from build123d import *

# Parameters (mm, degrees)
EXTRUDE_1_DEPTH              = 4
HOLE_WIZARD_M5_1_D           = 8
HOLE_WIZARD_M5_1_DEPTH       = 12.4
HOLE_WIZARD_M5_1_CBORE_D     = 9.5
HOLE_WIZARD_M5_1_CBORE_DEPTH = 0.9
HOLE_WIZARD_M5_1_TIP         = 2.403442476
SKETCH_4_R                   = 1.5
CUT_EXTRUDE_1_DEPTH          = 1
CUT_EXTRUDE_1_DEPTH_BACK     = 5


with BuildPart() as part:
    # 草图1 → 凸台-拉伸1 (new body)
    with BuildSketch(Plane(origin=(0, 0, 0), x_dir=(1, 0, 0), z_dir=(0, 1, 0))):
        with BuildLine():
            Line((0, 6.5), (30, 6.5))
            ThreePointArc((30, 6.5), (36.5, 0), (30, -6.5))
            Line((30, -6.5), (0, -6.5))
            ThreePointArc((0, -6.5), (-6.5, 0), (0, 6.5))
        make_face()
    extrude(amount=EXTRUDE_1_DEPTH)

    # M5 六角头螺栓的柱形沉头孔1
    with Locations(Plane(origin=(0, 4, 0), x_dir=(1, 0, 0), z_dir=(0, 1, 0))):
        with Locations((0, 0)):
            CounterBoreHole(HOLE_WIZARD_M5_1_D / 2, HOLE_WIZARD_M5_1_CBORE_D / 2, HOLE_WIZARD_M5_1_CBORE_DEPTH, depth=HOLE_WIZARD_M5_1_DEPTH)
            with Locations((0, 0, -(HOLE_WIZARD_M5_1_DEPTH + HOLE_WIZARD_M5_1_TIP / 2))):  # 118° drill point
                Cone(0, HOLE_WIZARD_M5_1_D / 2, HOLE_WIZARD_M5_1_TIP, mode=Mode.SUBTRACT)

    # 草图4 → 切除-拉伸1 (cut, two sides)
    with BuildSketch(Plane(origin=(0, 4, 0), x_dir=(1, 0, 0), z_dir=(0, 1, 0))) as cut_extrude_1_sk:
        with Locations((30, 0)):
            Circle(SKETCH_4_R)
    extrude(amount=CUT_EXTRUDE_1_DEPTH, mode=Mode.SUBTRACT)
    extrude(cut_extrude_1_sk.sketch, amount=-CUT_EXTRUDE_1_DEPTH_BACK, mode=Mode.SUBTRACT)


solid = part.part
The listing builds one solid part. Answer for the finished solid, in the listing's coordinates (mm). A direction names the side the tool comes from. Round coordinates to 2 decimals unless told otherwise and drop trailing zeros. Order: outer loops, then holes, each group sorted by start corner. A loop starts at its lowest first (then second) coordinate and runs counter-clockwise, first axis right, second up. Notation, with made-up numbers: M 56.5,22.5 L 80.5,22.5 A26 cw 80.5,41.5 Z; hole C -7,39.25 d5. An arc over 180 degrees is marked long. Answer in a Markdown table with one row per item. Add a question column.
1) Which of the six approach directions +Z, -Z, +X, -X, +Y, -Y give full straight-line access (tool end or side, diameter ignored) to faces 1 (the face through (-6.5, 2, 0.1)), 2 (the face through (2.192, 3.556, 4.214))?
2) The part is cut by section A-A on z = 0. Determine the outline of the cut face in (x, y).
3) Determine the mould class of faces 3 (the face through (28.5, 2.03, -0.07)), 4 (the face through (15, 2, -6.5)), 5 (the face through (15, 4, 0)) for opening direction Z: pulls with the +Z half, pulls with the -Z half, needs draft (parallel to the pull), parting line crosses it, or undercut.
4) The part is cut by section D-D on x = 0.5. Determine the outline of the cut face in (y, z), plus the area to 3 significant figures.
5) Flat-ended cylindrical pins translate along their axes: pin 1 Ø5 at (x, z) = (0, 0) entering from -Y; pin 2 Ø1.5 at (y, z) = (3, -2) entering from +X. Find the tip coordinate at first contact, or state that the pin passes through.
6) The part is cut by section C-C on z = -2.5. Determine the outline of the cut face in (x, y), plus the area to 3 significant figures.
7) The part is cut by section B-B on x = 29. Determine the outline of the cut face in (y, z).
8) Consider line 1 along Z through (x, y) = (30, 1.75); line 2 along Z through (x, y) = (0, 3.5); line 3 along X through (y, z) = (2.75, -0.5). Determine where each line is inside the solid, lowest interval first. Write a range as from..to.
Findings below:
| question | item | result |
|---|---|---|
| 1 | face 1 | -X, +Y, -Y |
| 1 | face 2 | +Y |
| 2 | outline | M -6.5,0 L -4,0 L -4,3.1 L -4.75,3.1 L -4.75,4 L -6.5,4 Z; M 4,0 L 28.5,0 L 28.5,4 L 4.75,4 L 4.75,3.1 L 4,3.1 Z; M 31.5,0 L 36.5,0 L 36.5,4 L 31.5,4 Z |
| 3 | face 3 | undercut |
| 3 | face 4 | pulls with the -Z half |
| 3 | face 5 | needs draft |
| 4 | outline | M 0,-6.5 L 4,-6.5 L 4,-4.72 L 3.1,-4.72 L 3.1,-3.97 L 0,-3.97 Z; M 0,3.97 L 3.1,3.97 L 3.1,4.72 L 4,4.72 L 4,6.5 L 0,6.5 Z |
| 4 | area | 18.9 mm² |
| 5 | pin 1 | passes through |
| 5 | pin 2 | stops at x = 36.38 |
| 6 | outline | M -6,0 L -3.12,0 L -3.12,3.1 L -4.04,3.1 L -4.04,4 L -6,4 Z; M 3.12,0 L 36,0 L 36,4 L 4.04,4 L 4.04,3.1 L 3.12,3.1 Z |
| 6 | area | 141 mm² |
| 7 | outline | M 0,-6.5 L 4,-6.5 L 4,-1.12 L 0,-1.12 Z; M 0,1.12 L 4,1.12 L 4,6.5 L 0,6.5 Z |
| 8 | line 1 | z = -6.5..-1.5, 1.5..6.5 |
| 8 | line 2 | z = -6.5..-4.75, 4.75..6.5 |
| 8 | line 3 | x = -6.48..-3.97, 3.97..28.59, 31.41..36.48 |
